Can you work these out from the drawing? Everything is in mm from the part's minimum corner. A direction names the side the tool comes from. Coordinates: 2 decimals unless noted, no trailing zeros. Loops run counter-clockwise (first coordinate to the right, second up) from the corner with the lowest first, then second, coordinate; pieces in that order, holes last. Notation, with made-up numbers: M 21,5.5 L 30,5.5 A16 cw 30,32.5 Z; hole C 55,2.25 d11. An arc over 180 degrees is marked long. Write each question's results on one line, items separated by ' | '.
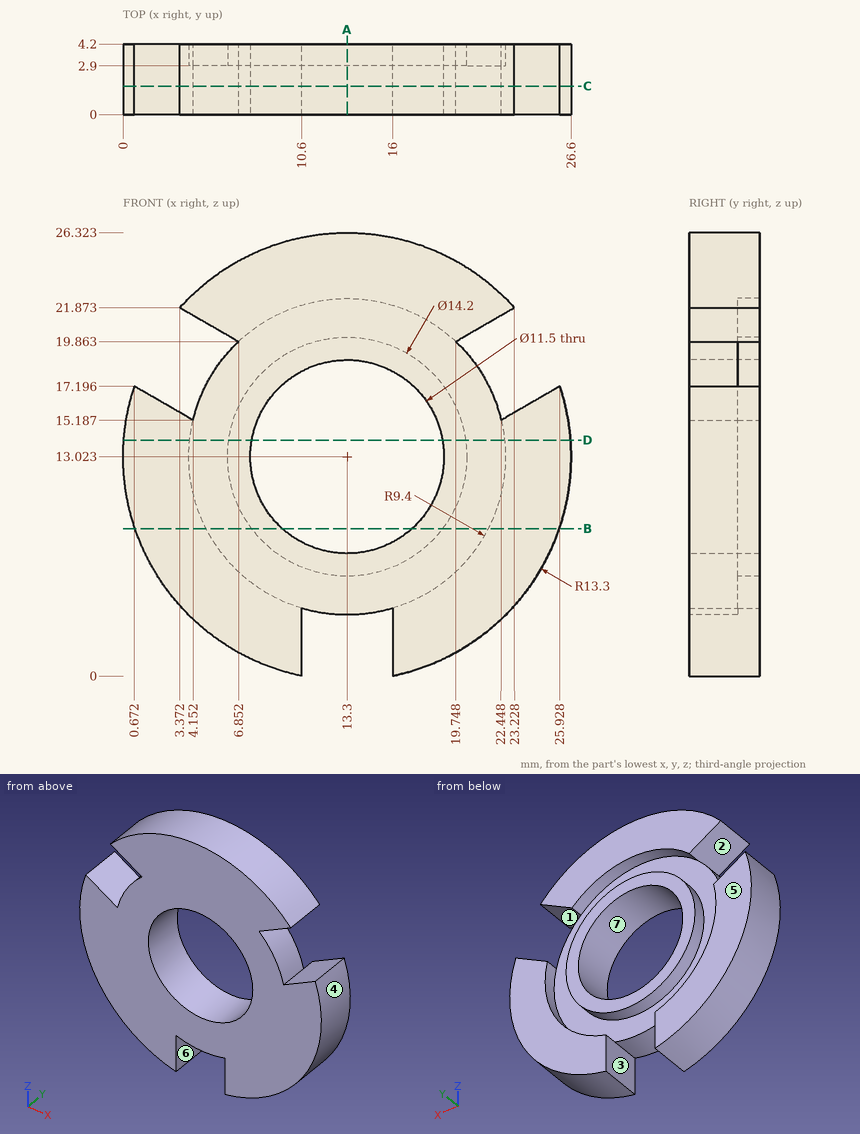
(1) If we mould it in two halves opening along X, with no side actions, what happens to the marked faces 4, 5, 6 and 7? For each: released by +X, released by -X, zero draft, split by the parting line, or undercut.
Reported:
face 4: released by +X | face 5: zero draft | face 6: undercut | face 7: undercut
(2) Please list where these lines run through material, in increasing order: probe 1 along Z at (x, y) = (13.3, 1.55); probe 2 along X at (y, z) = (3.9, 12) (1 decimal); probe 3 along Z at (x, y) = (13.3, 3.05). Write a range as from..to.
Reported:
probe 1: z = 3.62..7.27, 18.77..26.32 | probe 2: x = 0..4, 6.3..7.6, 19..20.3, 22.6..26.6 | probe 3: z = 5.92..7.27, 18.77..20.12, 22.42..26.32
(3) Imagine slicing it at D-D, the plane z = 14. List the corners of the cut face in (x, y) for me, and give its area (3 significant figures).
Reported:
outline: M 0.04,0 L 7.63,0 L 7.63,4.2 L 6.27,4.2 L 6.27,2.9 L 3.95,2.9 L 3.95,4.2 L 0.04,4.2 Z; M 18.97,0 L 26.56,0 L 26.56,4.2 L 22.65,4.2 L 22.65,2.9 L 20.33,2.9 L 20.33,4.2 L 18.97,4.2 Z | area: 57.8 mm2
(4) Will these pins go through, and if not, where does the flat tip stop? P1, Ø1.2, axis at y = 1.5, z = 2.5, coming from the +X side (1 decimal); P2, Ø2, axis at y = 3, z = 1.5, coming from the -X side (1 decimal); P3, Ø2, axis at x = 14.5, z = 3, coming from the +Y side; P4, Ø9, axis at x = 13.3, z = 13.02, coming from the -Y side.
Reported:
P1: stops at x = 22.2 | P2: stops at x = 5.2 | P3: stops at y = 2.9 | P4: passes through
(5) Imagine slicing it at B-B, the plane z = 8.75. List the corners of the cut face in (x, y) for me (1 decimal).
Reported:
outline: M 0.7,0 L 9.5,0 L 9.5,4.2 L 7.6,4.2 L 7.6,2.9 L 4.9,2.9 L 4.9,4.2 L 0.7,4.2 Z; M 17.1,0 L 25.9,0 L 25.9,4.2 L 21.7,4.2 L 21.7,2.9 L 19,2.9 L 19,4.2 L 17.1,4.2 Z
(6) Imagine slicing it at C-C, the plane y = 1.7. List the corners of the cut face in (x, z) for me, and give its area (3 significant figures).
Reported:
outline: M 0.67,17.2 A13.3 ccw 10.6,0 L 10.6,4.02 A9.4 ccw 16,4.02 L 16,0 A13.3 ccw 25.93,17.2 L 22.45,15.19 A9.4 ccw 19.75,19.86 L 23.23,21.87 A13.3 ccw 3.37,21.87 L 6.85,19.86 A9.4 ccw 4.15,15.19 Z; hole C 13.3,13.02 d11.5 | area: 388 mm2
(7) Imagine slicing it at A-A, the plane x = 13.3. List the corners of the cut face in (y, z) for me.
Reported:
outline: M 0,3.62 L 2.9,3.62 L 2.9,5.92 L 4.2,5.92 L 4.2,7.27 L 0,7.27 Z; M 0,18.77 L 4.2,18.77 L 4.2,20.12 L 2.9,20.12 L 2.9,22.42 L 4.2,22.42 L 4.2,26.32 L 0,26.32 Z
(8) Which directions (+Z, -Z, +X, -X, +Y, -Y) give clear straight access to the entire face, cutting with the end or side of a thin tool? Please do the marked faces 1, 2 and 3.
Reported:
face 1: +X, +Y, -Y | face 2: -X, +Y, -Y | face 3: -Z, +Y, -Y
